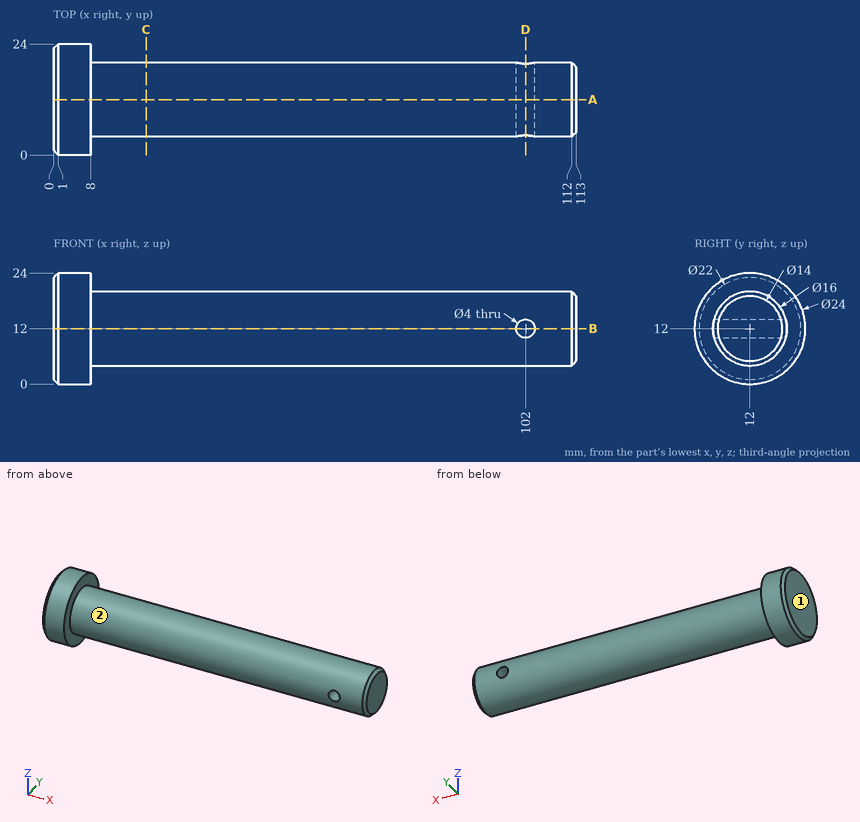
Input: dimensioned drawing with shaded views. Units: mm. Origin: part minimum x, y, z. A direction names the side the tool comes from. Round coordinates to 2 decimals unless told otherwise and drop trailing zeros. Write each loop counter-clockwise with the first axis right and the second up, starting at its lowest first coordinate (ties: lowest second). Pieces come first, ordered by that corner, then holes. Notation, with made-up numbers: (78, -25.75) -> (103, -25.75) arc R4 ccw to (103, -19.75) -> close; hole circle Ø5 at (11, 14). An arc over 180 degrees is marked (long way). Use CSV: the item, a comma, the result in double quotes. Start each with the question number.
Q1. Line query: L1, parallel to X at y = 16, z = 12; L2, parallel to Z at x = 102, y = 12.25; L3, parallel to X at y = 14, z = 21.5. Output: solid intervals per line, ascending.
Q2. First-contact query: pin 1 Ø1 at (y, z) = (20.5, 17.5) entering from +X; pin 2 Ø5 at (x, z) = (102, 12) entering from +Y; pin 3 Ø4 at (x, y) = (44, 9.5) entering from -Z; pin 4 Ø4 at (y, z) = (4.5, 19) entering from -X. Flat tips, straight axial feed; report the tip coordinate or a pass-through.
Q3. Reachability of the marked faces 1 and 2 from +Z, -Z, +X, -X, +Y, -Y: full face, straight path, thin tool, end or side. Return the list, or none.
Q4. Section C-C (x = 20). Return loops of the section in (y, z), plus the area to 3 significant figures.
Q5. Section A-A (y = 12). Return loops of the section in (x, z), plus the area to 3 significant figures.
Q6. Section B-B (z = 12). Return loops of the section in (x, y).
Q7. Section D-D (x = 102). Return loops of the section in (y, z).
Result sheet:
1,L1,"0 to 100, 104 to 113"
1,L2,"4 to 10, 14 to 20"
1,L3,"0 to 8"
2,pin 1,"x = 8"
2,pin 2,"y = 20"
2,pin 3,"z = 4.02"
2,pin 4,"x = 0"
3,face 1,"+Z, -Z, -X, +Y, -Y"
3,face 2,"+X"
4,outline,"circle Ø16 at (12, 12)"
4,area,"201 mm²"
5,outline,"(0, 1) -> (1, 0) -> (8, 0) -> (8, 4) -> (112, 4) -> (113, 5) -> (113, 19) -> (112, 20) -> (8, 20) -> (8, 24) -> (1, 24) -> (0, 23) -> close; hole circle Ø4 at (102, 12)"
5,area,"1,860 mm²"
6,outline,"(0, 1) -> (1, 0) -> (8, 0) -> (8, 4) -> (100, 4) -> (100, 20) -> (8, 20) -> (8, 24) -> (1, 24) -> (0, 23) -> close; (104, 4) -> (112, 4) -> (113, 5) -> (113, 19) -> (112, 20) -> (104, 20) -> close"
7,outline,"(4.25, 10) arc R8 ccw to (19.75, 10) -> close; (4.25, 14) -> (19.75, 14) arc R8 ccw to start"
